Build history of the part. All positions in model axes, mm. Face numbers are marked on the shaded views. A direction names the side the tool comes from. Give positions to 0.01 mm unless a question says otherwise; leave off trailing zeros. Write each loop counter-clockwise with the first axis right and the second up, starting at its lowest first coordinate (ties: lowest second). Pieces come first, ordered by that corner, then holes. Notation, with made-up numbers: M -10.5,23 L 8.5,23 A18 cw 8.5,51 Z; hole C -10,-19 d1. An arc over 180 degrees is marked long. Return JSON: item names as keys, results as strings. Group by question number.
Q1. Band-saw the part on A-A, the plane y = -2.25. Give the cut face in (x, z) (3 decimals), then the cut area to 3 significant figures.
Q2. Tool access for the marked faces 1 and 2: list every direction of +Z, -Z, +X, -X, +Y, -Y with a clear straight run to the whole face (end or side of a thin tool).
Q3. Band-saw the part on C-C, the plane z = 1.25. Give the cut face in (x, y), then the cut area to 3 significant figures.
Q4. Band-saw the part on B-B, the plane x = -4.5. Give the cut face in (y, z) (3 decimals), then the cut area to 3 significant figures.
Q5. Wall check: probe 1 along Y at (x, z) = (-1, 1.85); probe 2 along Y at (x, z) = (-7.5, 1.8); probe 3 along Y at (x, z) = (8, 1.5). Give the ranges that are in metal, low to high.
Q6. Pull direction X, two halves, no side cores. Call the marked faces 3, 4 and 5: +X half, -X half, draft (parallel to the pull), parting line (faces both ways), or undercut.
from build123d import *

# Parameters (mm, degrees)
SKETCH2_W           = 22.6822
SKETCH2_H           = 18.034
SKETCH2_R           = 1.3462
SKETCH2_W_2         = 9.9822
SKETCH2_H_2         = 5.334
BOSS_EXTRUDE1_DEPTH = 3.175


with BuildPart() as part:
    # Sketch2 → Boss-Extrude1 (new body)
    with BuildSketch(Plane.XY):
        Rectangle(SKETCH2_W, SKETCH2_H)
        with Locations((-7.112, 5.334)):
            Circle(SKETCH2_R, mode=Mode.SUBTRACT)
        with Locations(Location((7.112, 5.334, 0), (0, 0, 180))):
            Circle(SKETCH2_R, mode=Mode.SUBTRACT)
        with Locations((7.112, -5.334)):
            Circle(SKETCH2_R, mode=Mode.SUBTRACT)
        with Locations(Location((-7.112, -5.334, 0), (0, 0, 180))):
            Circle(SKETCH2_R, mode=Mode.SUBTRACT)
        Rectangle(SKETCH2_W_2, SKETCH2_H_2, mode=Mode.SUBTRACT)
    extrude(amount=BOSS_EXTRUDE1_DEPTH)


solid = part.part
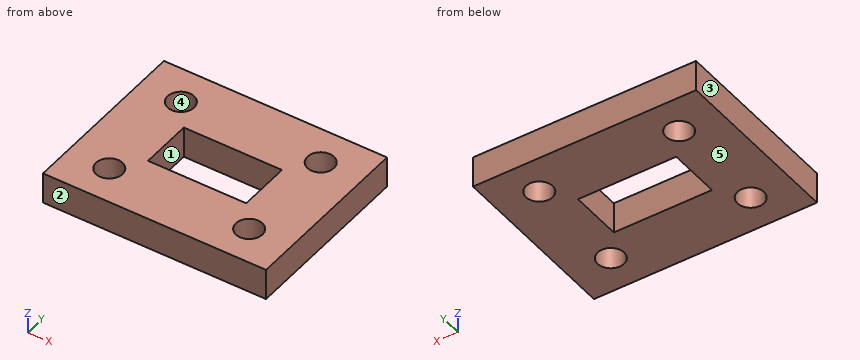
From the geometry:
{
 "1": {"outline": "M -11.341,0 L -4.991,0 L -4.991,3.175 L -11.341,3.175 Z; M 4.991,0 L 11.341,0 L 11.341,3.175 L 4.991,3.175 Z", "area": "40.3 mm^2"},
 "2": {"face 1": "+Z, -Z", "face 2": "+Z, -Z, +X, -X, -Y"},
 "3": {"outline": "M -11.34,-9.02 L 11.34,-9.02 L 11.34,9.02 L -11.34,9.02 Z; hole C -7.11,-5.33 d2.69; hole C -7.11,5.33 d2.69; hole M -4.99,-2.67 L 4.99,-2.67 L 4.99,2.67 L -4.99,2.67 Z; hole C 7.11,-5.33 d2.69; hole C 7.11,5.33 d2.69", "area": "333 mm^2"},
 "4": {"outline": "M -9.017,0 L -2.667,0 L -2.667,3.175 L -9.017,3.175 Z; M 2.667,0 L 9.017,0 L 9.017,3.175 L 2.667,3.175 Z", "area": "40.3 mm^2"},
 "5": {"probe 1": "y = -9.02 to -2.67, 2.67 to 9.02", "probe 2": "y = -9.02 to -6.62, -4.04 to 4.04, 6.62 to 9.02", "probe 3": "y = -9.02 to -6.35, -4.32 to 4.32, 6.35 to 9.02"},
 "6": {"face 3": "-X half", "face 4": "undercut", "face 5": "draft"}
}
